The model under review builds one solid part; all positions refer to its coordinate system, in mm. A direction names the side the tool comes from. Round coordinates to 2 decimals unless told otherwise and drop trailing zeros. Write each loop counter-clockwise with the first axis right and the second up, starting at its lowest first coordinate (ties: lowest second). Pieces come first, ordered by that corner, then holes. Notation, with made-up numbers: (29, 29.25) -> (56, 29.25) arc R24 ccw to (56, 57.25) -> close; hole circle Ø2 at (-30.75, -12). An arc over 180 degrees is marked (long way). Return JSON: item names as keys, results as strings. Group by question number.
1. Take a section at B-B, the plane x = 0. Write out the cut boundary in (y, z).
2. Take a section at D-D, the plane y = 3.5. Write out the cut boundary in (x, z), then the cut area to 3 significant figures.
3. Clearance check with flat-ended pins moving along their axes: P1, Ø0.8, axis at x = -1, y = 13.5, coming from the +Z side; P2, Ø0.6, axis at x = -0.5, y = 13.5, coming from the -Z side; P3, Ø3, axis at x = 0, z = 1.5, coming from the -Y side. State where each tip first meets the part, or that it passes through.
4. Take a section at C-C, the plane y = 12.25. Write out the cut boundary in (x, z).
5. Tool access review of faces 1 (the cylindrical face through (1.5, 5.93, 0.07)), 2 (the flat face through (0, 0, 0)): name each direction out of +Z, -Z, +X, -X, +Y, -Y from which nothing blocks a thin tool from reaching the whole face with its end or side.
6. Take a section at A-A, the plane z = 0. Write out the cut boundary in (x, y).
7. For line 1 along Y through (x, z) = (1.3, 1.5); line 2 along X through (y, z) = (11.5, 0); line 3 along Z through (x, y) = (-0.75, 10.25), list the stretches that pass through material, from the lowest coordinate up. Write a range as from..to.
Autodesk Inventor part; units mm, degrees
ref_plane "YZ Plane" through (0, 0, 0) normal (1, 0, 0) x (0, 1, 0)
ref_plane "XZ Plane" through (0, 0, 0) normal (0, 1, 0) x (-1, 0, 0)
ref_plane "XY Plane" through (0, 0, 0) normal (0, 0, 1) x (1, 0, 0)
sketch "Sketch1" plane through (0, 0, 0) normal (0, 0, 1) x (1, 0, 0)
  line L0 (0, 0) -> (-1.5, 0)
  line L1 (-1.5, 0) -> (-1.5, 11)
  line L2 (-1.5, 11) -> (-1.5, 11)
  line L3 (-1.5, 11) -> (-1.5, 12)
  line L4 (-1.5, 12) -> (-3, 12)
  line L5 (-3, 12) -> (-3, 14)
  line L6 (-3, 14) -> (0, 14)
  line L7 (0, 14) -> (0, 0)
  dimension "d0" = 2
  dimension "d1" = 3
  dimension "d2" = 1.5
  dimension "d3" = 0
  dimension "d4" = 1
  dimension "d5" = 14
  dimension "d6" = 90
revolve "Revolution1" add sketch "Sketch1" angle 360 about axis through (0, 14, 0) along (0, -1, 0)
thread "Thread1"
sketch "Sketch2" plane through (0, 14, 0) normal (0, 1, 0) x (1, 0, 0)
  line L0 (5, 0.35) -> (-5, 0.35)
  line L1 (-5, 0.35) -> (-5, -0.35)
  line L2 (-5, -0.35) -> (5, -0.35)
  line L3 (5, -0.35) -> (5, 0.35)
  line L4 (5, 0.35) -> (-5, -0.35) construction
  line L5 (-5, 0.35) -> (5, -0.35) construction
  point P0 (0, 0)
  dimension "d10" = 10
  dimension "d11" = 0.7
fillet "Fillet1" radius 0.25 1 edges at (3, 14, 0)
extrude "Extrusion2" cut sketch "Sketch2" against normal blind 0.7
fillet "Fillet2" radius 0.3 1 edges at (1.5, 12, 0)
properties part number "TorsionOscillator-Screw-M3-Brass-CheeseHead-12mm-Std" material "Brass, Soft Yellow"
Output:
{
 "1": {"outline": "(0, -1.5) -> (11.7, -1.5) arc R0.3 cw to (12, -1.8) -> (12, -3) -> (13.75, -3) arc R0.25 ccw to (14, -2.75) -> (14, -0.35) -> (13.3, -0.35) -> (13.3, 0.35) -> (14, 0.35) -> (14, 2.75) arc R0.25 ccw to (13.75, 3) -> (12, 3) -> (12, 1.8) arc R0.3 cw to (11.7, 1.5) -> (0, 1.5) -> close"},
 "2": {"outline": "circle Ø3 at (0, 0)", "area": "7.07 mm^2"},
 "3": {"P1": "stops at z = 2.94", "P2": "stops at z = -2.99", "P3": "stops at y = 0"},
 "4": {"outline": "circle Ø6 at (0, 0)"},
 "5": {"face 1": "-Y", "face 2": "+Z, -Z, +X, -X, -Y"},
 "6": {"outline": "(-3, 12) -> (-1.8, 12) arc R0.3 cw to (-1.5, 11.7) -> (-1.5, 0) -> (1.5, 0) -> (1.5, 11.7) arc R0.3 cw to (1.8, 12) -> (3, 12) -> (3, 13.3) -> (-3, 13.3) -> close"},
 "7": {"line 1": "y = 12..14", "line 2": "x = -1.5..1.5", "line 3": "z = -1.3..1.3"}
}
